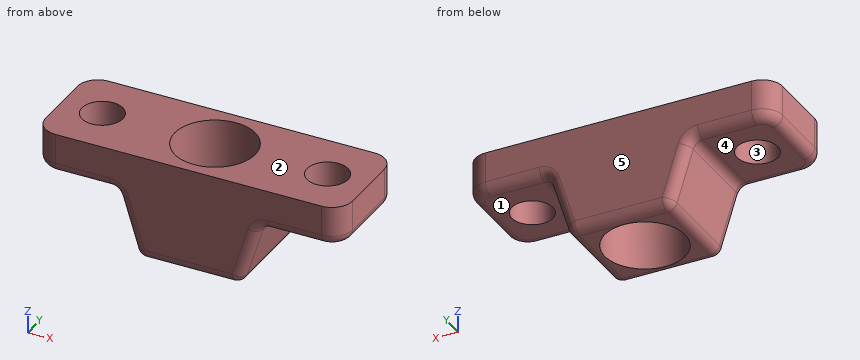
from build123d import *

# Parameters (mm, degrees)
BOSS_EXTRUDE1_DEPTH = 12.7
SKETCH2_R           = 5
CUT_EXTRUDE1_DEPTH  = 14.137790614
SKETCH3_R           = 2.54
CUT_EXTRUDE2_DEPTH  = 6
FILLET1_R           = 2.54
FILLET2_R           = 1.27


with BuildPart() as part:
    # Sketch1 → Boss-Extrude1 (new body)
    with BuildSketch(Plane(origin=(0, 0, 0), x_dir=(1, 0, 0), z_dir=(0, 1, 0))):
        Polygon((19.05, 0), (-19.05, 0), (-19.05, 5), (-8.89, 5), (-6.35, 13.137790614), (6.35, 13.137790614), (8.89, 5), (19.05, 5), align=None)
    extrude(amount=BOSS_EXTRUDE1_DEPTH)

    # Sketch2 → Cut-Extrude1 (cut, through all)
    with BuildSketch(Plane(origin=(0, 0, -13.137790614), x_dir=(-1, 0, 0), z_dir=(0, 0, -1))):
        with Locations((0, 6.35)):
            Circle(SKETCH2_R)
    extrude(amount=-CUT_EXTRUDE1_DEPTH, mode=Mode.SUBTRACT)

    # Sketch3 → Cut-Extrude2 (cut, through all)
    with BuildSketch(Plane(origin=(0, 0, -5), x_dir=(-1, 0, 0), z_dir=(0, 0, -1))):
        with Locations((13.97, 6.35)):
            Circle(SKETCH3_R)
        with Locations((-13.97, 6.35)):
            Circle(SKETCH3_R)
    extrude(amount=-CUT_EXTRUDE2_DEPTH, mode=Mode.SUBTRACT)

    # Fillet1
    fillet1_edges = [part.edges().sort_by_distance(p)[0] for p in [
        (19.05, 12.7, -2.5),
        (-19.05, 0, -2.5),
        (-19.05, 12.7, -2.5),
        (19.05, 0, -2.5),
    ]]
    fillet(fillet1_edges, radius=FILLET1_R)

    # Fillet2
    fillet2_edges = [part.edges().sort_by_distance(p)[0] for p in [
        (-8.89, 6.35, -5),
        (-6.35, 6.35, -13.137790614),
        (6.35, 6.35, -13.137790614),
        (8.89, 6.35, -5),
        (7.62, 12.7, -9.068895307),
        (0, 12.7, -13.137790614),
        (-7.62, 12.7, -9.068895307),
        (-12.7, 12.7, -5),
        (-19.05, 6.35, -5),
        (12.7, 0, -5),
        (-18.306051224, 11.956051224, -5),
        (-18.306051224, 0.743948776, -5),
        (19.05, 6.35, -5),
        (12.7, 12.7, -5),
        (18.306051224, 11.956051224, -5),
        (18.306051224, 0.743948776, -5),
        (-12.7, 0, -5),
        (-7.62, 0, -9.068895307),
        (0, 0, -13.137790614),
        (7.62, 0, -9.068895307),
    ]]
    fillet(fillet2_edges, radius=FILLET2_R)


solid = part.part
Verification items for the finished model (mm, model axes). Face numbers are marked on the shaded views. A direction names the side the tool comes from. Give positions to 0.01 mm unless a question says otherwise; leave off trailing zeros. Order: outer loops, then holes, each group sorted by start corner. A loop starts at its lowest first (then second) coordinate and runs counter-clockwise, first axis right, second up. Notation, with made-up numbers: M 1.25,-26 L 46.25,-26 A28 cw 46.25,6 Z; hole C -15.5,-31.5 d9. An arc over 180 degrees is marked long. Answer as a JSON object with one key per item and string values. Group by question number.
1) Scan lines: line 1 along Y through (x, z) = (13.97, -2.85); line 2 along Z through (x, y) = (-10, 11.5); line 3 along X through (y, z) = (4.75, -4). Record each from-to range of solid material in increasing order. Write a range as [from, to].
2) Access from +Z, -Z, +X, -X, +Y, -Y to the whole of each face (thin tool, end or side, straight path). Record for the marked faces 1 and 2.
3) Cross-section at B-B (z = -2). Enter the section's corners in (x, y).
4) Mould release check, pull along Y, two halves, no side actions. Record for the marked faces 3, 4 and 5: released by +Y, released by -Y, zero draft, split by the parting line, or undercut.
5) Depth check by flat-ended pin: pin 1 Ø3 at (x, y) = (-13.97, 6.35) entering from +Z; pin 2 Ø1 at (x, z) = (-4.5, -10.5) entering from -Y; pin 3 Ø2.5 at (x, y) = (12.5, 5) entering from -Z. Enter the tip coordinate at first touch or a pass-through.
6) Cross-section at D-D (x = 0). Enter the section's corners in (y, z).
7) Cross-section at C-C (y = 6.35). Enter the section's corners in (x, z).
8) Cross-section at A-A (x = -4). Enter the section's corners in (y, z).
Result sheet:
{
 "1": {"line 1": "y = [0, 3.81], [8.89, 12.7]", "line 2": "z = [-5, 0]", "line 3": "x = [-19.02, -15.94], [-12, -4.74], [4.74, 12], [15.94, 19.02]"},
 "2": {"face 1": "-Z, +X, +Y, -Y", "face 2": "+Z, +X, -X, +Y, -Y"},
 "3": {"outline": "M -19.05,2.54 A2.54 ccw -16.51,0 L 16.51,0 A2.54 ccw 19.05,2.54 L 19.05,10.16 A2.54 ccw 16.51,12.7 L -16.51,12.7 A2.54 ccw -19.05,10.16 Z; hole C -13.97,6.35 d5.08; hole C 0,6.35 d10; hole C 13.97,6.35 d5.08"},
 "4": {"face 3": "undercut", "face 4": "zero draft", "face 5": "released by +Y"},
 "5": {"pin 1": "passes through", "pin 2": "stops at y = 0", "pin 3": "stops at z = -5"},
 "6": {"outline": "M 0,-11.87 A1.27 ccw 1.27,-13.14 L 1.35,-13.14 L 1.35,0 L 0,0 Z; M 11.35,-13.14 L 11.43,-13.14 A1.27 ccw 12.7,-11.87 L 12.7,0 L 11.35,0 Z"},
 "7": {"outline": "M -19.05,-3.73 A1.27 ccw -17.78,-5 L -16.51,-5 L -16.51,0 L -19.05,0 Z; M -11.43,-5 L -9.82,-5 A1.27 cw -8.61,-5.89 L -6.63,-12.25 A1.27 ccw -5.42,-13.14 L -5,-13.14 L -5,0 L -11.43,0 Z; M 5,-13.14 L 5.42,-13.14 A1.27 ccw 6.63,-12.25 L 8.61,-5.89 A1.27 cw 9.82,-5 L 11.43,-5 L 11.43,0 L 5,0 Z; M 16.51,-5 L 17.78,-5 A1.27 ccw 19.05,-3.73 L 19.05,0 L 16.51,0 Z"},
 "8": {"outline": "M 0,-11.87 A1.27 ccw 1.27,-13.14 L 3.35,-13.14 L 3.35,0 L 0,0 Z; M 9.35,-13.14 L 11.43,-13.14 A1.27 ccw 12.7,-11.87 L 12.7,0 L 9.35,0 Z"}
}
